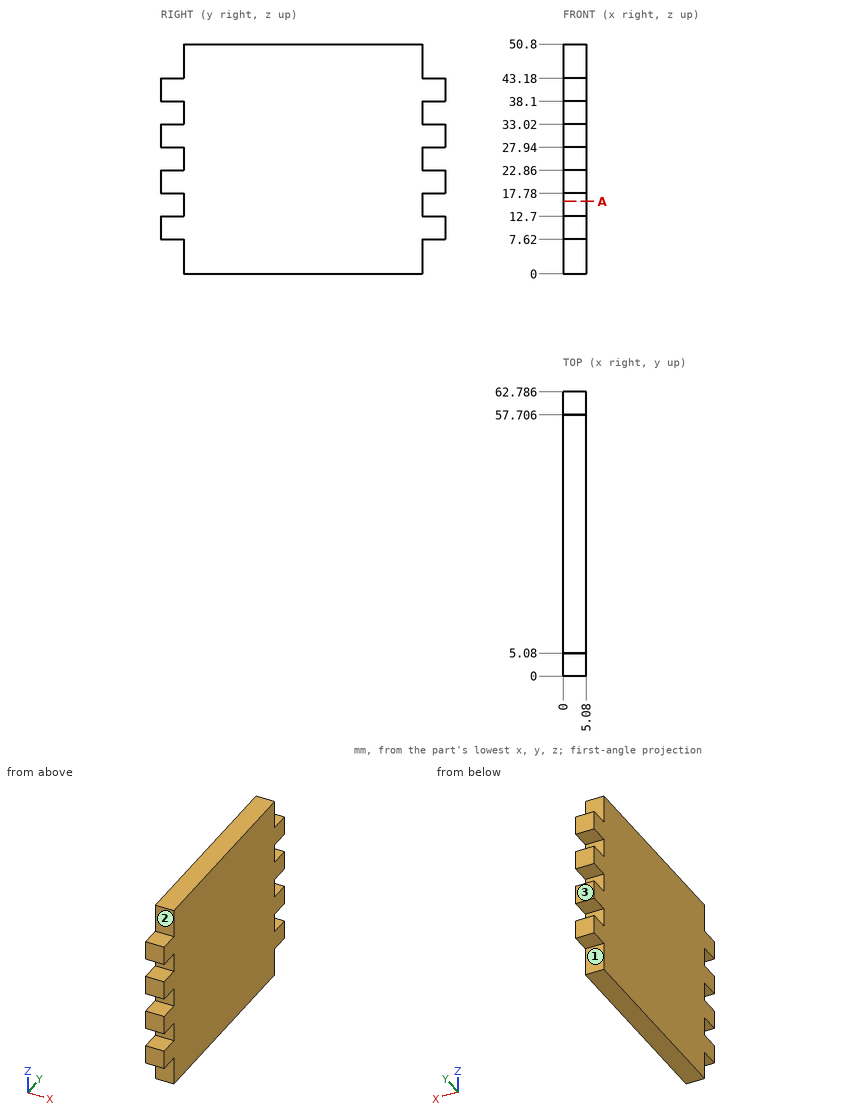
The figure shows three views and two pictorial views of one solid part (mm, origin at its lowest corner). Answer the questions. A direction names the side the tool comes from. Give positions to 0.01 mm unless a question says otherwise; leave off trailing zeros. Loops run counter-clockwise (first coordinate to the right, second up) from the corner with the lowest first, then second, coordinate; pieces in that order, holes last. Notation, with made-up numbers: (-8, 65) - (8, 65) arc R21 cw to (8, 78) - close; hole circle Ø9 at (-1.5, 25). An arc over 180 degrees is marked (long way). Answer in a Markdown table with one row per item.
(1) Section A-A (z = 16) is taken. Give the vertices of the cut face in (x, y).
Results list:
| item | result |
|---|---|
| outline | (0, 5.08) - (5.08, 5.08) - (5.08, 57.71) - (0, 57.71) - close |
(2) Flat-ended cylindrical pins translate along their axes: pin 1 Ø1.5 at (x, z) = (3, 2.5) entering from +Y; pin 2 Ø1.5 at (x, y) = (2, 59.5) entering from -Z; pin 3 Ø2.5 at (x, y) = (2, 59) entering from +Z. Find the tip coordinate at first contact, or state that the pin passes through.
Results list:
| item | result |
|---|---|
| pin 1 | stops at y = 57.71 |
| pin 2 | stops at z = 7.62 |
| pin 3 | stops at z = 43.18 |
(3) Consider L1, parallel to Z at x = 2.2, y = 60; L2, parallel to Y at x = 0.35, z = 25.5. Determine where each line is inside the solid, lowest interval first. Write a range as [from, to].
Results list:
| item | result |
|---|---|
| L1 | z = [7.62, 12.7], [17.78, 22.86], [27.94, 33.02], [38.1, 43.18] |
| L2 | y = [5.08, 57.71] |
(4) A tool of negligible diameter and unlimited length cuts with its end or side. For the marked faces 1, 2 and 3, from which of +Z, -Z, +X, -X, +Y, -Y can it reach the whole face along a straight path? Write none if from no direction.
Results list:
| item | result |
|---|---|
| face 1 | -Z, +X, -X, +Y |
| face 2 | +Z, +X, -X, -Y |
| face 3 | +Z, -Z, +X, -X, +Y |
